Autodesk Inventor part; units mm, degrees
ref_plane "YZ Plane" through (0, 0, 0) normal (1, 0, 0) x (0, 1, 0)
ref_plane "XZ Plane" through (0, 0, 0) normal (0, 1, 0) x (-1, 0, 0)
ref_plane "XY Plane" through (0, 0, 0) normal (0, 0, 1) x (1, 0, 0)
sketch "Boceto3" plane through (0, 0, 0) normal (1, 0, 0) x (0, 1, 0)
  line L0 (0, -90) -> (0, -91)
  line L1 (0, -91) -> (10, -91)
  line L2 (10, -91) -> (10, -77)
  line L3 (-3.586, -60.6037) -> (-3.586, -77) construction
  line L4 (-3.586, -77) -> (10, -77) construction
  spline S0 degree 2 poles (-3.586, -60.6037) (-3.586, -77) (10, -77) knots 1 1 1 2 2 2
  line L5 (0, 0) -> (10, 0)
  line L6 (10, 0) -> (10, -17)
  line L7 (10, -17) -> (-3.586, -37.9742) construction
  line L8 (-3.586, -37.9742) -> (-3.586, -60.6037) construction
  spline S1 degree 2 poles (10, -17) (-3.586, -37.9742) (-3.586, -60.6037) knots 1 1 1 2 2 2
  line L9 (0, -91) -> (-10, -91) construction
  line L10 (-10, -91) -> (-10, -81) construction
  spline S2 degree 2 poles (0, -91) (-10, -91) (-10, -81) knots 1 1 1 2 2 2
  line L11 (-3.586, -76) -> (-2.6, -76)
  circle A0 centre (-2.6, -76) radius 2.6
  circle A1 centre (0.9686, -25.3255) radius 2.6
  line L12 (0, 0) -> (0, -17) construction
  line L13 (0, -17) -> (-5.2, -20.5234) construction
  spline S3 degree 2 poles (0, 0) (0, -17) (-5.2, -20.5234) knots 1 1 1 2 2 2
  line L14 (-5.2, -20.5234) -> (-10, -81)
  dimension "d36" = 1
  dimension "d40" = 10
  dimension "d41" = 17
extrude "Extrusión4" add sketch "Boceto3" against normal blind 9
fillet "Empalme1" radius 2 1 edges at (-4.5, -5.2, -20.5234)
fillet "Empalme2" radius 2 1 edges at (-4.5, 0, 0)
sketch "Boceto4" plane through (0, 10, -77) normal (0, 1, 0) x (1, 0, 0)
  line L0 (0, 14) -> (0, 0)
  line L1 (0, 14) -> (-4.5, 14)
  line L2 (0, 14) -> (-9, 14)
  point P0 (0, -77)
sketch "Boceto5" plane through (0, 10, 0) normal (0, 1, 0) x (1, 0, 0)
  point P0 (0, 0)
sketch "Boceto7" plane through (0, 10, -77) normal (0, 1, 0) x (1, 0, 0)
  line L0 (0, 14) -> (-9, 14)
  line L1 (-4.5, 14) -> (-4.5, 7)
  circle A0 centre (-4.5, 7) radius 3.25
  line L2 (-4.5, 7) -> (-4.5, -66.8)
  circle A1 centre (-4.5, -66.8) radius 3.25
  point P0 (0, -77)
  dimension "d67" = 7
  dimension "d68" = 6.5
  dimension "d69" = 73.8
  dimension "d70" = 6.5
extrude "Extrusión7" cut sketch "Boceto7" against normal blind 20
sketch "Boceto8" plane through (-9, -10, -81) normal (0, -0.9969, 0.0791) x (1, 0, 0)
  point P0 (9, 81.5373)
sketch "Boceto9" plane through (0, 10, 0) normal (0, 1, 0) x (1, 0, 0)
  point P0 (0, 0)
CAD build for the part. Positions are in the model's coordinates, mm. Round coordinates to 2 decimals unless told otherwise and drop trailing zeros.
Item 1: Probe line 1 along X through (y, z) = (0.5, -84); line 2 along Z through (x, y) = (-7.5, 7.5); line 3 along Z through (x, y) = (-0.75, 9). List the from-to ranges inside material, lowest first.
Item 2: Pin check, flat tips, straight feed: pin 1 (4 mm diameter, centred on x = -1.5, z = -46.5, fed in from +Y); pin 2 (3 mm diameter, centred on x = -4.5, z = -46.5, fed in from -Y); pin 3 (5 mm diameter, centred on x = -4.5, y = -7, fed in from -Z); pin 4 (4 mm diameter, centred on y = -2.6, z = -76, fed in from -X). Stop position of each tip, or through.
Item 3: Mould opens along X. For faces 1 (the face through (-9, -2.4, -44.9)), 2 (the face through (-4.437, 0.405, -27.864)), 3 (the face through (-5.205, 0.14, -80.827)) say: pulls with the +X half, pulls with the -X half, needs draft (parallel to the pull), parting line crosses it, or undercut.
Item 4: Saw through at A-A on y = -2.6. State how many separate pieces and enclosed holes the cut face has, then the cut area to 3 significant figures.
Reported:
1. line 1: x = -9 to -7.75, -1.25 to 0
1. line 2: z = -91 to -85.25, -82.75 to -76.85, -21.07 to -11.45, -8.95 to 0
1. line 3: z = -91 to -76.98, -18.58 to 0
2. pin 1: stops at y = -1.82
2. pin 2: stops at y = -7.38
2. pin 3: stops at z = -90.33
2. pin 4: passes through
3. face 1: pulls with the -X half
3. face 2: needs draft
3. face 3: undercut
4. separate pieces: 3
4. enclosed holes: 1
4. area: 404 mm2
